The model under review builds one solid part; all positions refer to its coordinate system, in mm. Round coordinates to 2 decimals unless told otherwise and drop trailing zeros. Write each loop counter-clockwise with the first axis right and the second up, starting at its lowest first coordinate (ties: lowest second). Pieces come first, ordered by that corner, then holes.
Item 1: Clearance check with flat-ended pins moving along their axes: pin 1 Ø12 at (y, z) = (7, 2) entering from +X; pin 2 Ø2.5 at (x, z) = (36.5, -20.5) entering from -Y; pin 3 Ø0.6 at (x, y) = (36.5, 7) entering from +Z. State where each tip first meets the part, or that it passes through.
Item 2: Add section B-B (y = 21). Give the boundary of the cut face in (x, z).
Item 3: Add section A-A (z = 14). Give the boundary of the cut face in (x, y).
Item 4: To check wall thickness, follow L1, parallel to X at y = 6.5, z = 15; L2, parallel to Z at x = -9, y = 22.25; L3, parallel to X at y = 23.75, z = -18. State the ranges of each line that lie inside material, in increasing order.
```python
from build123d import *

# Parameters (mm, degrees)
SKETCH1_W           = 70
SKETCH1_H           = 55
BOSS_EXTRUDE1_DEPTH = 25
FILLET1_R           = 3
SKETCH2_W           = 3.300925217
SKETCH2_H           = 1.959924347
BOSS_EXTRUDE2_DEPTH = 3
SKETCH3_R           = 0.719628756
CUT_EXTRUDE1_DEPTH  = 22


with BuildPart() as part:
    # Sketch1 → Boss-Extrude1 (new body)
    with BuildSketch(Plane(origin=(0, 0, 0), x_dir=(1, 0, 0), z_dir=(0, 1, 0))):
        Rectangle(SKETCH1_W, SKETCH1_H)
    extrude(amount=BOSS_EXTRUDE1_DEPTH)

    # Fillet1
    fillet1_edges = [part.edges().sort_by_distance(p)[0] for p in [
        (-35, 25, 0),
        (0, 25, 27.5),
        (35, 25, 0),
        (0, 0, 27.5),
        (-35, 0, 0),
        (0, 0, -27.5),
        (35, 0, 0),
        (35, 12.5, 27.5),
        (-35, 12.5, 27.5),
        (-35, 12.5, -27.5),
        (35, 12.5, -27.5),
        (0, 25, -27.5),
    ]]
    fillet(fillet1_edges, radius=FILLET1_R)

    # Sketch2 → Boss-Extrude2 (add)
    with BuildSketch(Plane(origin=(35, 0, 0), x_dir=(0, 0, -1), z_dir=(1, 0, 0))):
        with Locations((20.501840212, 17.399810869)):
            Rectangle(SKETCH2_W, SKETCH2_H)
        with Locations((20.604994125, 6.87811174)):
            Rectangle(SKETCH2_W, SKETCH2_H)
    extrude(amount=BOSS_EXTRUDE2_DEPTH)

    # Sketch3 → Cut-Extrude1 (cut)
    with BuildSketch(Plane(origin=(0, 18.379773042, 0), x_dir=(1, 0, 0), z_dir=(0, 1, 0))):
        with Locations(Location((36.345846873, 20.613426823, 0), (0, 0, 270))):
            Circle(SKETCH3_R)
    extrude(amount=-CUT_EXTRUDE1_DEPTH, mode=Mode.SUBTRACT)


solid = part.part
```
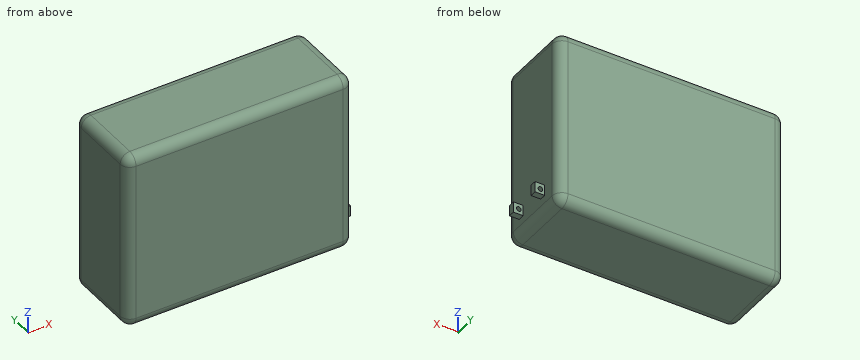
Numbers:
1. pin 1: stops at x = 35
1. pin 2: stops at y = 5.9
1. pin 3: stops at z = -18.95
2. outline: (-35, -24.5) arc R3 ccw to (-32, -27.5) - (32, -27.5) arc R3 ccw to (35, -24.5) - (35, 24.5) arc R3 ccw to (32, 27.5) - (-32, 27.5) arc R3 ccw to (-35, 24.5) - close
3. outline: (-35, 3) arc R3 ccw to (-32, 0) - (32, 0) arc R3 ccw to (35, 3) - (35, 22) arc R3 ccw to (32, 25) - (-32, 25) arc R3 ccw to (-35, 22) - close
4. L1: x = -35 to 35
4. L2: z = -27.49 to 27.49
4. L3: x = -34.44 to 34.44
